Autodesk Inventor part; units mm, degrees
ref_plane "YZ Plane" through (0, 0, 0) normal (1, 0, 0) x (0, 1, 0)
ref_plane "XZ Plane" through (0, 0, 0) normal (0, 1, 0) x (-1, 0, 0)
ref_plane "XY Plane" through (0, 0, 0) normal (0, 0, 1) x (1, 0, 0)
sketch "Boceto1" plane through (0, 0, 0) normal (0, 0, 1) x (1, 0, 0)
  circle A0 centre (0, 0) radius 57.15
  circle A1 centre (101.6, 0) radius 44.45
  circle A2 centre (-31.75, 47.519) radius 11.1125
  circle A3 centre (-31.75, -47.519) radius 11.1125
  circle A4 centre (114.3, 42.5971) radius 11.1125
  circle A5 centre (114.3, -42.5971) radius 11.1125
  line L0 (7.1437, 56.7018) -> (107.1562, 44.1014)
  circle A6 centre (44.45, 52.0016) radius 11.1125
  line L1 (7.1437, -56.7018) -> (107.1562, -44.1014)
  circle A7 centre (44.45, -52.0016) radius 11.1125
  dimension "d0" = 114.3
  dimension "d1" = 88.9
  dimension "d2" = 203.2
  dimension "d3" = 22.225
  dimension "d4" = 22.225
  dimension "d7" = 22.225
  dimension "d8" = 22.225
  dimension "d11" = 22.225
  dimension "d13" = 0
  dimension "d14" = 22.225
  dimension "d27" = 12.7
  dimension "d28" = 12.7
  dimension "d29" = 44.45
  dimension "d30" = 44.45
  dimension "d31" = 31.75
  dimension "d32" = 31.75
extrude "Extrusión1" add sketch "Boceto1" along normal blind 4.445
sketch "Boceto2" plane through (0, 0, 4.445) normal (0, 0, 1) x (1, 0, 0)
  arc A0 (-21.9537, 52.7651) -> (-40.3458, 40.4764) centre (-31.75, 47.519) ccw
  circle A1 centre (-31.75, 47.519) radius 4.2164
  arc A2 (-40.3458, -40.4764) -> (-21.9537, -52.7651) centre (-31.75, -47.519) ccw
  circle A3 centre (-31.75, -47.519) radius 4.2164
  arc A4 (33.4247, -53.3907) -> (55.4753, -50.6125) centre (44.45, -52.0016) ccw
  circle A5 centre (44.45, -52.0016) radius 4.2164
  arc A6 (55.4753, 50.6125) -> (33.4247, 53.3907) centre (44.45, 52.0016) ccw
  circle A7 centre (44.45, 52.0016) radius 4.2164
  arc A8 (124.4689, 38.1158) -> (103.3657, 44.5789) centre (114.3, 42.5971) ccw
  circle A9 centre (114.3, 42.5971) radius 4.2164
  arc A10 (103.3657, -44.5789) -> (124.4689, -38.1158) centre (114.3, -42.5971) ccw
  circle A11 centre (114.3, -42.5971) radius 4.2164
  point P0 (0, 0)
  dimension "d18" = 8.4328
  dimension "d19" = 8.4328
  dimension "d20" = 8.4328
  dimension "d21" = 8.4328
  dimension "d22" = 8.4328
  dimension "d23" = 8.4328
extrude "Extrusión2" cut sketch "Boceto2" against normal up to surface (4.445 mm away)
fillet "Empalme1" radius 6.35 12 edges at (-21.9537, -52.7651, 2.2225) (-40.3458, -40.4764, 2.2225) (33.4247, -53.3907, 2.2225) (55.4753, -50.6125, 2.2225) (124.4689, -38.1158, 2.2225) (-40.3458, 40.4764, 2.2225) (-21.9537, 52.7651, 2.2225) (33.4247, 53.3907, 2.2225) (55.4753, 50.6125, 2.2225) (103.3657, 44.5789, 2.2225) (124.4689, 38.1158, 2.2225) (103.3657, -44.5789, 2.2225)
sketch "Boceto3" plane through (0, 0, 0) normal (0, 0, -1) x (-1, 0, 0)
  circle A0 centre (0, 0) radius 7.1437
  circle A1 centre (0, -45) radius 6
  circle A2 centre (0, 45) radius 6
  line L0 (0, -45) -> (0, 0)
  line L1 (0, 0) -> (0, 45)
  dimension "d33" = 14.2875
  dimension "d34" = 12
  dimension "d35" = 12
  dimension "d36" = 45
  dimension "d37" = 45
extrude "Extrusión3" cut sketch "Boceto3" against normal up to surface (4.445 mm away)
equation "\"d16\" = t"
equation "\"d18\" = Q"
equation "\"d19\" = Q"
equation "\"d20\" = Q"
equation "\"d21\" = Q"
equation "\"d22\" = Q"
equation "\"d23\" = Q"
equation "\"d33\" = DF"
equation "\"d34\" = NF"
equation "\"d35\" = NF"
equation "\"t\" = 4.445"
equation "\"Q\" = 8.4328"
equation "\"DF\" = 14.2875"
equation "\"NF\" = 12"
properties part number "STEEL SIDE REDUCTION COUNTER PLATE"
Geometry check sheet. Reference: the model listing, model coordinates, mm. A direction names the side the tool comes from. Coordinates: 2 decimals unless noted, no trailing zeros. Order: outer loops, then holes, each group sorted by start corner. A loop starts at its lowest first (then second) coordinate and runs counter-clockwise, first axis right, second up. Notation, with made-up numbers: (-29.5, 19.25) - (12.5, 19.25) arc R16 ccw to (12.5, 24.25) - close; hole circle Ø1 at (57.5, 67.25). An arc over 180 degrees is marked (long way). One line per item, written item: value.
(1) Depth check by flat-ended pin: pin 1 Ø11 at (x, y) = (44.45, 52) entering from +Z (3 decimals); pin 2 Ø2 at (y, z) = (-44.5, 2) entering from -X; pin 3 Ø6.5 at (x, y) = (114.3, -42.6) entering from +Z; pin 4 Ø1.5 at (x, z) = (-15, 3) entering from -Y. Enter the tip coordinate at first touch or a pass-through.
Data:
pin 1: stops at z = 4.445
pin 2: stops at x = -42.68
pin 3: passes through
pin 4: stops at y = -55.34
(2) Sectioned sample at A-A (x = 114.3). Enter the section's corners in (y, z) (1 decimal).
Data:
outline: (-53.7, 0) - (-46.8, 0) - (-46.8, 4.4) - (-53.7, 4.4) - close; (-38.4, 0) - (38.4, 0) - (38.4, 4.4) - (-38.4, 4.4) - close; (46.8, 0) - (53.7, 0) - (53.7, 4.4) - (46.8, 4.4) - close
(3) Access from +Z, -Z, +X, -X, +Y, -Y to the whole of each face (thin tool, end or side, straight path). Record for faces 1 (the face through (41.3, -49.2, 2.3)), 2 (the face through (57.134, 51.549, 2.254)), 3 (the face through (79.27, -47.615, 2.191)).
Data:
face 1: +Z, -Z
face 2: +Z, -Z, +Y
face 3: +Z, -Z, -Y
(4) Sectioned sample at C-C (x = -31.75). Enter the section's corners in (y, z) (1 decimal).
Data:
outline: (-58.6, 0) - (-51.7, 0) - (-51.7, 4.4) - (-58.6, 4.4) - close; (-43.3, 0) - (43.3, 0) - (43.3, 4.4) - (-43.3, 4.4) - close; (51.7, 0) - (58.6, 0) - (58.6, 4.4) - (51.7, 4.4) - close
(5) Thickness scan on probe 1 along Y at (x, z) = (-31.75, 1.55); probe 2 along Y at (x, z) = (0, 2.1); probe 3 along Y at (x, z) = (44.45, 3.35). Record the ranges inside material, lowest first. Write a range as from..to.
Data:
probe 1: y = -58.63..-51.74, -43.3..43.3, 51.74..58.63
probe 2: y = -57.15..-51, -39..-7.14, 7.14..39, 51..57.15
probe 3: y = -63.11..-56.22, -47.79..47.79, 56.22..63.11
(6) Sectioned sample at B-B (y = 0). Enter the section's corners in (x, z) (3 decimals).
Data:
outline: (-57.15, 0) - (-7.144, 0) - (-7.144, 4.445) - (-57.15, 4.445) - close; (7.144, 0) - (146.05, 0) - (146.05, 4.445) - (7.144, 4.445) - close
(7) Sectioned sample at D-D (y = -31). Enter the section's corners in (x, z) (3 decimals), and give its area (3 significant figures).
Data:
outline: (-48.012, 0) - (133.456, 0) - (133.456, 4.445) - (-48.012, 4.445) - close
area: 807 mm^2
(8) Release check for a two-part mould opening along Y. For faces 4 (the face through (1.301, -50.857, 2.191)), 5 (the face through (17.579, 55.387, 2.191)), 6 (the face through (116.246, -46.338, 2.254)), 7 (the face through (57.21, -51.48, 2.25)) record: +Y half, -Y half, draft (parallel to the pull), parting line (faces both ways), or undercut.
Data:
face 4: undercut
face 5: +Y half
face 6: undercut
face 7: -Y half
